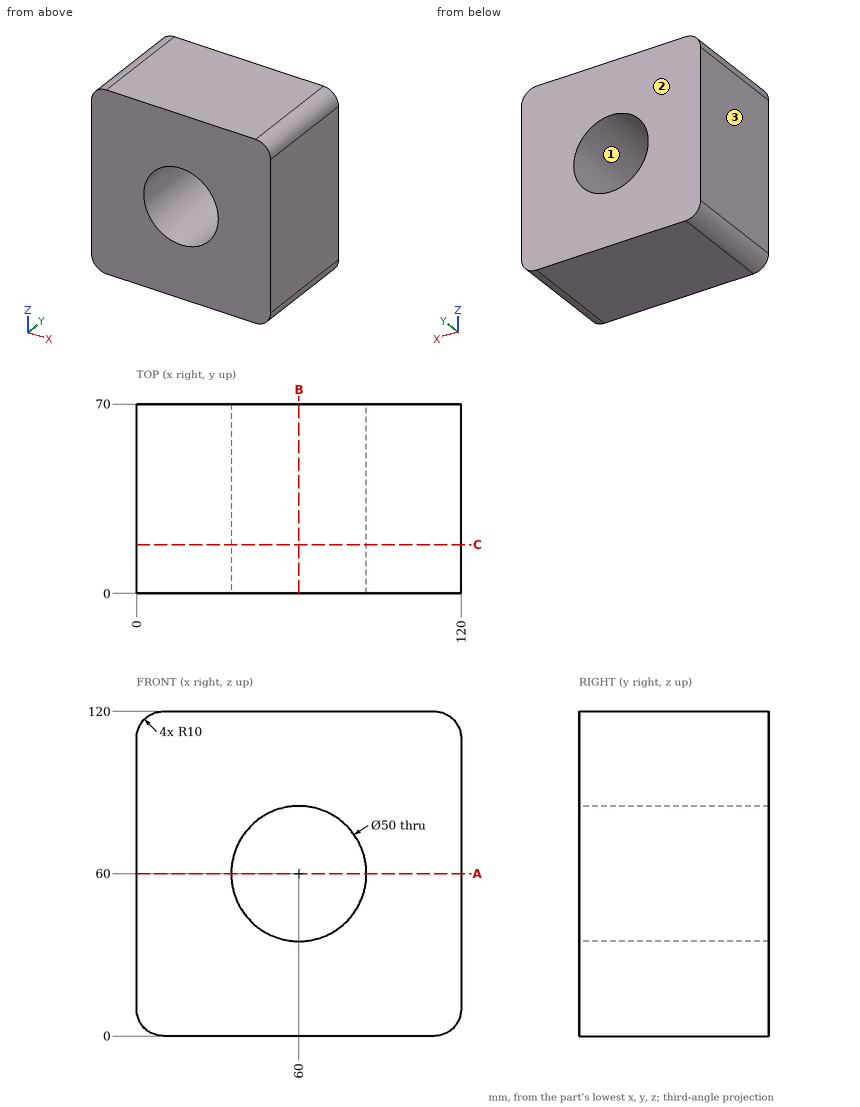
Here's the drawing with two shaded views (mm, measured from the low corner). I have some questions. Round coordinates to 2 decimals unless told otherwise and drop trailing zeros. Write each loop counter-clockwise with the first axis right and the second up, starting at its lowest first coordinate (ties: lowest second). Pieces come first, ordered by that corner, then holes. Notation, with made-up numbers: M 84,19 L 102,19 A17 ccw 102,49 Z; hole C -36,62 d8. An arc over 180 degrees is marked long. Answer in a Markdown table with one row per item. Add a question column.
Q1. Imagine slicing it at C-C (y = 18). Please give me the cut outline in (x, z).
Q2. Imagine slicing it at A-A (z = 60). Please give me the cut outline in (x, y).
Q3. If we mould it in two halves opening along X, with no side actions, what happens to the marked faces 1, 2 and 3? For each: +X half, -X half, draft (parallel to the pull), parting line (faces both ways), or undercut.
Q4. Imagine slicing it at B-B (x = 60). Please give me the cut outline in (y, z).
Q5. If I drill on line 1 (Z direction, x = 60, y = 40); line 2 (Z direction, x = 82, y = 55.5); line 3 (X direction, y = 44.5, z = 45), over which ranges is the centre line in solid material (lowest first)? Write a range as from..to.
Values:
| question | item | result |
|---|---|---|
| 1 | outline | M 0,10 A10 ccw 10,0 L 110,0 A10 ccw 120,10 L 120,110 A10 ccw 110,120 L 10,120 A10 ccw 0,110 Z; hole C 60,60 d50 |
| 2 | outline | M 0,0 L 35,0 L 35,70 L 0,70 Z; M 85,0 L 120,0 L 120,70 L 85,70 Z |
| 3 | face 1 | undercut |
| 3 | face 2 | draft |
| 3 | face 3 | -X half |
| 4 | outline | M 0,0 L 70,0 L 70,35 L 0,35 Z; M 0,85 L 70,85 L 70,120 L 0,120 Z |
| 5 | line 1 | 0..35, 85..120 |
| 5 | line 2 | 0..48.13, 71.87..120 |
| 5 | line 3 | 0..40, 80..120 |
